Check sheet for the modelled part. Datum: model origin and axes. Units: mm. Coordinates: 2 decimals unless noted, no trailing zeros. Write each loop counter-clockwise with the first axis right and the second up, starting at its lowest first coordinate (ties: lowest second). Pieces come first, ordered by that corner, then holes. Notation, with made-up numbers: (50, 75) - (72, 75) arc R24 cw to (72, 95) - close; hole circle Ø5 at (40.5, 47.5). An arc over 180 degrees is marked (long way). Use one line per item in the form item = value. Start each with the question number.
1. Cross-section at B-B on x = -4.5. Record the boundary of the cut face in (y, z), then the cut area to 3 significant figures.
2. Cross-section at C-C on z = 8.75. Record the boundary of the cut face in (x, y), then the cut area to 3 significant figures.
3. Scan lines: line 1 along Z through (x, y) = (4.25, -14.5); line 2 along Z through (x, y) = (3.75, -5); line 3 along X through (y, z) = (-15.75, -8.75). Record each from-to range of solid material in increasing order.
4. Cross-section at A-A on y = -15.5. Record the boundary of the cut face in (x, z).
```python
from build123d import *

# Parameters (mm, degrees)
SRECTANGLE_W     = 10
SRECTANGLE_H     = 20
FRECTANGLE_DEPTH = 20
FRRECTANGLE_R    = 2


with BuildPart() as part:
    # SRectangle → FRectangle (new body)
    with BuildSketch(Plane(origin=(0, 0, 0), x_dir=(1, 0, 0), z_dir=(0, 1, 0))):
        Rectangle(SRECTANGLE_W, SRECTANGLE_H)
    extrude(amount=-FRECTANGLE_DEPTH)

    # FRRectangle
    frrectangle_edges = [part.edges().sort_by_distance(p)[0] for p in [
        (5, -10, 10),
        (-5, -10, 10),
        (-5, -10, -10),
        (5, -10, -10),
    ]]
    fillet(frrectangle_edges, radius=FRRECTANGLE_R)


solid = part.part
```
Final values:
q1.outline = (-20, -9.32) - (0, -9.32) - (0, 9.32) - (-20, 9.32) - close
q1.area = 373 mm²
q2.outline = (-4.85, -20) - (4.85, -20) - (4.85, 0) - (-4.85, 0) - close
q2.area = 194 mm²
q3.line_1 = -9.56 to 9.56
q3.line_2 = -9.85 to 9.85
q3.line_3 = -4.85 to 4.85
q4.outline = (-5, -8) arc R2 ccw to (-3, -10) - (3, -10) arc R2 ccw to (5, -8) - (5, 8) arc R2 ccw to (3, 10) - (-3, 10) arc R2 ccw to (-5, 8) - close
